from build123d import *

# Parameters (mm, degrees)
SKETCH1_W               = 49.5
SKETCH1_H               = 61.5
BOSS_EXTRUDE1_DEPTH     = 23.75
SKETCH2_W               = 46
SKETCH2_H               = 58
CUT_EXTRUDE1_DEPTH      = 22
SKETCH3_W               = 3
SKETCH3_H               = 16
CUT_EXTRUDE2_DEPTH      = 1.75
SKETCH7_W               = 3
SKETCH7_H               = 5
BOSS_EXTRUDE2_DEPTH     = 6
SKETCH11_W              = 37.5
SKETCH11_H              = 61.5
BOSS_EXTRUDE3_DEPTH     = 15
SKETCH12_W              = 34.5
SKETCH12_H              = 57
CUT_EXTRUDE3_DEPTH      = 15
SKETCH14_W              = 7.75
SKETCH14_H              = 9
BOSS_EXTRUDE4_DEPTH     = 0.0001
SKETCH15_W              = 4.15
SKETCH15_H              = 5.2
CUT_EXTRUDE4_DEPTH      = 4.75
SKETCH16_W              = 8.5
SKETCH16_H              = 15.5
BOSS_EXTRUDE5_DEPTH     = 16.75
SKETCH17_W              = 5.125
SKETCH17_H              = 6.625
CUT_EXTRUDE5_DEPTH      = 8.5
CUT_EXTRUDE6_DEPTH      = 15
CUT_EXTRUDE6_DEPTH_BACK = 1.75
SKETCH18_W              = 5
SKETCH18_H              = 12
SKETCH20_W              = 16
SKETCH20_H              = 4.5
CUT_EXTRUDE7_DEPTH      = 1.75
SKETCH21_W              = 32.25
SKETCH21_H              = 81.5
BOSS_EXTRUDE7_DEPTH     = 10
SKETCH23_W              = 28.75
SKETCH23_H              = 78
CUT_EXTRUDE8_DEPTH      = 10
SKETCH25_W              = 3
SKETCH25_H              = 5.4
BOSS_EXTRUDE8_DEPTH     = 1.75
SKETCH28_W              = 3
SKETCH28_H              = 2
BOSS_EXTRUDE9_DEPTH     = 1.75
SKETCH30_W              = 5
SKETCH30_H              = 1.5
BOSS_EXTRUDE11_DEPTH    = 1
SKETCH32_W              = 10.5
SKETCH32_H              = 2.25
CUT_EXTRUDE9_DEPTH      = 1.75
SKETCH33_W              = 11
SKETCH33_H              = 11
CUT_EXTRUDE10_DEPTH     = 1
SKETCH34_W              = 11
SKETCH34_H              = 1
BOSS_EXTRUDE12_DEPTH    = 2
SKETCH35_W              = 19
SKETCH35_H              = 10
CUT_EXTRUDE11_DEPTH     = 1.75
SKETCH36_W              = 1.75
SKETCH36_H              = 21.5
CUT_EXTRUDE12_DEPTH     = 5.75
SKETCH37_W              = 7.5
SKETCH37_H              = 7.5
SKETCH37_W_2            = 28.75
BOSS_EXTRUDE13_DEPTH    = 1.75


with BuildPart() as part:
    # Sketch1 → Boss-Extrude1 (new body)
    with BuildSketch(Plane(origin=(0, 0, 0), x_dir=(1, 0, 0), z_dir=(0, 1, 0))):
        with Locations((-113.412024913, -45.391200727)):
            Rectangle(SKETCH1_W, SKETCH1_H)
    extrude(amount=BOSS_EXTRUDE1_DEPTH)

    # Sketch2 → Cut-Extrude1 (cut)
    with BuildSketch(Plane(origin=(0, 0, 0), x_dir=(-1, 0, 0), z_dir=(0, -1, 0))):
        with Locations((113.412024913, -45.391200727)):
            Rectangle(SKETCH2_W, SKETCH2_H)
    extrude(amount=-CUT_EXTRUDE1_DEPTH, mode=Mode.SUBTRACT)

    # Sketch3 → Cut-Extrude2 (cut)
    with BuildSketch(Plane(origin=(0, 22, 0), x_dir=(-1, 0, 0), z_dir=(0, -1, 0))):
        with Locations((91.912024913, -66.391200727)):
            Rectangle(SKETCH3_W, SKETCH3_H)
        with Locations((91.912024913, -24.391200727)):
            Rectangle(SKETCH3_W, SKETCH3_H)
        with Locations((91.912024913, -45.391200727)):
            Rectangle(SKETCH3_W, SKETCH3_H)
    extrude(amount=-CUT_EXTRUDE2_DEPTH, mode=Mode.SUBTRACT)

    # Sketch7 → Boss-Extrude2 (add)
    with BuildSketch(Plane(origin=(0, 22, 0), x_dir=(-1, 0, 0), z_dir=(0, -1, 0))):
        with Locations((91.912024913, -55.891200727)):
            Rectangle(SKETCH7_W, SKETCH7_H)
        with Locations((91.912024913, -34.891200727)):
            Rectangle(SKETCH7_W, SKETCH7_H)
    extrude(amount=BOSS_EXTRUDE2_DEPTH)

    # Sketch11 → Boss-Extrude3 (add)
    with BuildSketch(Plane(origin=(0, 23.75, 0), x_dir=(1, 0, 0), z_dir=(0, 1, 0))):
        with Locations((-119.412024913, -45.391200727)):
            Rectangle(SKETCH11_W, SKETCH11_H)
    extrude(amount=BOSS_EXTRUDE3_DEPTH)

    # Sketch12 → Cut-Extrude3 (cut)
    with BuildSketch(Plane(origin=(0, 38.75, 0), x_dir=(1, 0, 0), z_dir=(0, 1, 0))):
        with Locations((-119.412024913, -45.391200727)):
            Rectangle(SKETCH12_W, SKETCH12_H)
    extrude(amount=-CUT_EXTRUDE3_DEPTH, mode=Mode.SUBTRACT)

    # Sketch14 → Boss-Extrude4 (add)
    with BuildSketch(Plane(origin=(0, 23.75, 0), x_dir=(1, 0, 0), z_dir=(0, 1, 0))):
        with Locations((-92.542024913, -66.391200727)):
            Rectangle(SKETCH14_W, SKETCH14_H)
    extrude(amount=BOSS_EXTRUDE4_DEPTH)

    # Sketch15 → Cut-Extrude4 (cut)
    with BuildSketch(Plane(origin=(0, 23.7501, 0), x_dir=(1, 0, 0), z_dir=(0, 1, 0))):
        with Locations((-92.542024913, -66.391200727)):
            Rectangle(SKETCH15_W, SKETCH15_H)
    extrude(amount=-CUT_EXTRUDE4_DEPTH, mode=Mode.SUBTRACT)

    # Sketch16 → Boss-Extrude5 (add)
    with BuildSketch(Plane(origin=(0, 23.75, 0), x_dir=(1, 0, 0), z_dir=(0, 1, 0))):
        with Locations((-92.912024913, -24.391200727)):
            Rectangle(SKETCH16_W, SKETCH16_H)
    extrude(amount=BOSS_EXTRUDE5_DEPTH)

    # Sketch17 → Cut-Extrude5 (cut)
    with BuildSketch(Plane(origin=(-88.662024913, 0, 0), x_dir=(0, 0, -1), z_dir=(1, 0, 0))):
        with Locations((-27.828700727, 35.4375)):
            Rectangle(SKETCH17_W, SKETCH17_H)
        with Locations((-27.828700727, 27.0625)):
            Rectangle(SKETCH17_W, SKETCH17_H)
        with Locations((-20.953700727, 35.4375)):
            Rectangle(SKETCH17_W, SKETCH17_H)
        with Locations((-20.953700727, 27.0625)):
            Rectangle(SKETCH17_W, SKETCH17_H)
    extrude(amount=-CUT_EXTRUDE5_DEPTH, mode=Mode.SUBTRACT)

    # Sketch18 → Cut-Extrude6 (cut, two sides: drawn at the far end of the back side and taken through both)
    with BuildSketch(Plane(origin=(0, 23.75, 0), x_dir=(1, 0, 0), z_dir=(0, 1, 0)).offset(-CUT_EXTRUDE6_DEPTH_BACK)):
        with Locations((-92.912024913, -24.391200727)):
            Rectangle(SKETCH18_W, SKETCH18_H)
    extrude(amount=CUT_EXTRUDE6_DEPTH + CUT_EXTRUDE6_DEPTH_BACK, mode=Mode.SUBTRACT)

    # Sketch20 → Cut-Extrude7 (cut)
    with BuildSketch(Plane(origin=(-100.662024913, 0, 0), x_dir=(0, 0, -1), z_dir=(1, 0, 0))):
        with Locations((-45.391200727, 26)):
            Rectangle(SKETCH20_W, SKETCH20_H)
    extrude(amount=-CUT_EXTRUDE7_DEPTH, mode=Mode.SUBTRACT)

    # Sketch21 → Boss-Extrude7 (add)
    with BuildSketch(Plane(origin=(0, 0, 0), x_dir=(-1, 0, 0), z_dir=(0, -1, 0))):
        with Locations((152.537024913, -45.391200727)):
            Rectangle(SKETCH21_W, SKETCH21_H)
    extrude(amount=-BOSS_EXTRUDE7_DEPTH)

    # Sketch23 → Cut-Extrude8 (cut)
    with BuildSketch(Plane(origin=(0, 10, 0), x_dir=(1, 0, 0), z_dir=(0, 1, 0))):
        with Locations((-152.537024913, -45.391200727)):
            Rectangle(SKETCH23_W, SKETCH23_H)
    extrude(amount=-CUT_EXTRUDE8_DEPTH, mode=Mode.SUBTRACT)

    # Sketch25 → Boss-Extrude8 (add)
    with BuildSketch(Plane(origin=(0, 22, 0), x_dir=(-1, 0, 0), z_dir=(0, -1, 0))):
        with Locations((91.912024913, -61.091200727)):
            Rectangle(SKETCH25_W, SKETCH25_H)
        with Locations((91.912024913, -71.691200727)):
            Rectangle(SKETCH25_W, SKETCH25_H)
    extrude(amount=-BOSS_EXTRUDE8_DEPTH)

    # Sketch28 → Boss-Extrude9 (add)
    with BuildSketch(Plane(origin=(0, 23.75, 0), x_dir=(1, 0, 0), z_dir=(0, 1, 0))):
        with Locations((-91.912024913, -17.391200727)):
            Rectangle(SKETCH28_W, SKETCH28_H)
        with Locations((-91.912024913, -31.391200727)):
            Rectangle(SKETCH28_W, SKETCH28_H)
    extrude(amount=-BOSS_EXTRUDE9_DEPTH)

    # Sketch30 → Boss-Extrude11 (add)
    with BuildSketch(Plane.ZY.offset(93.412024913)):
        with Locations((55.891200727, 16.75)):
            Rectangle(SKETCH30_W, SKETCH30_H)
        with Locations((34.891200727, 16.75)):
            Rectangle(SKETCH30_W, SKETCH30_H)
    extrude(amount=BOSS_EXTRUDE11_DEPTH)

    # Sketch32 → Cut-Extrude9 (cut)
    with BuildSketch(Plane(origin=(0, 38.75, 0), x_dir=(1, 0, 0), z_dir=(0, 1, 0))):
        with Locations((-119.412024913, -75.016200727)):
            Rectangle(SKETCH32_W, SKETCH32_H)
        with Locations((-119.412024913, -15.766200727)):
            Rectangle(SKETCH32_W, SKETCH32_H)
    extrude(amount=-CUT_EXTRUDE9_DEPTH, mode=Mode.SUBTRACT)

    # Sketch33 → Cut-Extrude10 (cut)
    with BuildSketch(Plane.ZY.offset(90.412024913)):
        with Locations((32.891200727, 5.5)):
            Rectangle(SKETCH33_W, SKETCH33_H)
    extrude(amount=-CUT_EXTRUDE10_DEPTH, mode=Mode.SUBTRACT)

    # Sketch34 → Boss-Extrude12 (add)
    with BuildSketch(Plane.ZY.offset(90.412024913)):
        with Locations((32.891200727, 11.5)):
            Rectangle(SKETCH34_W, SKETCH34_H)
        Polygon((38.391200727, 12), (38.391200727, 11), (38.391200727, 0), (39.391200727, 0), (39.391200727, 12), align=None)
        Polygon((26.391200727, 0), (27.391200727, 0), (27.391200727, 11), (27.391200727, 12), (26.391200727, 12), align=None)
    extrude(amount=BOSS_EXTRUDE12_DEPTH)

    # Sketch35 → Cut-Extrude11 (cut)
    with BuildSketch(Plane(origin=(0, 0, 14.641200727), x_dir=(-1, 0, 0), z_dir=(0, 0, -1))):
        with Locations((123.412024913, 5)):
            Rectangle(SKETCH35_W, SKETCH35_H)
    extrude(amount=-CUT_EXTRUDE11_DEPTH, mode=Mode.SUBTRACT)

    # Sketch36 → Cut-Extrude12 (cut)
    with BuildSketch(Plane(origin=(0, 0, 0), x_dir=(-1, 0, 0), z_dir=(0, -1, 0))):
        with Locations((137.287024913, -45.391200727)):
            Rectangle(SKETCH36_W, SKETCH36_H)
    extrude(amount=-CUT_EXTRUDE12_DEPTH, mode=Mode.SUBTRACT)

    # Sketch37 → Boss-Extrude13 (add)
    with BuildSketch(Plane(origin=(0, 0, 0), x_dir=(-1, 0, 0), z_dir=(0, -1, 0))):
        with Locations((94.162024913, -70.641200727)):
            Rectangle(SKETCH37_W, SKETCH37_H)
        with Locations((94.162024913, -20.141200727)):
            Rectangle(SKETCH37_W, SKETCH37_H)
        with Locations((152.537024913, -70.641200727)):
            Rectangle(SKETCH37_W_2, SKETCH37_H)
        with Locations((152.537024913, -20.141200727)):
            Rectangle(SKETCH37_W_2, SKETCH37_H)
    extrude(amount=-BOSS_EXTRUDE13_DEPTH)


solid = part.part
For this review, take the finished solid that the model builds, in its own axes (mm). A direction names the side the tool comes from. Give positions to 0.01 mm unless a question says otherwise; leave off trailing zeros. Order: outer loops, then holes, each group sorted by start corner. A loop starts at its lowest first (then second) coordinate and runs counter-clockwise, first axis right, second up. Notation, with made-up numbers: (12, -29.75) - (49, -29.75) arc R11 cw to (49, -24.75) - close; hole circle Ø7 at (-37, 64). An arc over 180 degrees is marked (long way). Answer as a JSON object with one key per item and string values. Group by question number.
Item 1: Clearance check with flat-ended pins moving along their axes: pin 1 Ø4.5 at (y, z) = (30.5, 26.5) entering from -X; pin 2 Ø3 at (x, z) = (-126, 22.5) entering from +Y; pin 3 Ø12 at (x, z) = (-137, 67.5) entering from +Y. State where each tip first meets the part, or that it passes through.
Item 2: Take a section at C-C on z = 45. Give the boundary of the cut face in (x, y).
Item 3: Wall thickness on line 1 along X through (y, z) = (8, 36); line 2 along X through (y, z) = (2, 60.5); line 3 along Y through (x, z) = (-97, 21.5) (3 decimals): over which ranges is each line inside the solid? List them lowest first.
Item 4: Take a section at B-B on y = 26. Give the boundary of the cut face in (x, z).
Item 5: Machinability: for faces 4 (the flat face through (-89.412, 6, 33)), 5 (the flat face through (-95, 23.75, 66)), 6 (the flat face through (-102, 38.75, 45)), which of the approach directions +Z, -Z, +X, -X, +Y, -Y give a long, thin tool a straight path to every point of the face, cutting with its end or side? Answer none if there is none.
Item 6: Take a section at A-A on y = 35. Give the boundary of the cut face in (x, z), and give its area (3 significant figures).
Item 7: Draft analysis for pull direction Y (two halves, no side actions). For faces 1 (the flat face through (-92, 19, 32.391)), 2 (the flat face through (-136.412, 11, 46)), 3 (the flat face through (-137, 0, 60)), state which applies: pulls with the +Y half, pulls with the -Y half, needs draft (parallel to the pull), parting line crosses it, or undercut.
Item 8: Take a section at D-D on x = -156. Give the boundary of the cut face in (y, z).
Reported:
{
 "1": {"pin 1": "x = -138.16", "pin 2": "y = 23.75", "pin 3": "y = 38.75"},
 "2": {"outline": "(-168.66, 0) - (-166.91, 0) - (-166.91, 10) - (-168.66, 10) - close; (-138.16, 5.75) - (-136.41, 5.75) - (-136.41, 22) - (-93.41, 22) - (-93.41, 23.75) - (-136.66, 23.75) - (-136.66, 38.75) - (-138.16, 38.75) - close; (-102.16, 28.25) - (-100.66, 28.25) - (-100.66, 38.75) - (-102.16, 38.75) - close; (-90.41, 0) - (-88.66, 0) - (-88.66, 23.75) - (-90.41, 23.75) - close"},
 "3": {"line 1": "-168.66 to -166.91, -138.16 to -136.41, -89.41 to -88.66", "line 2": "-168.66 to -166.91, -138.16 to -136.41, -90.41 to -88.66", "line 3": "0 to 1.75, 22 to 23.75, 30.375 to 32.125, 38.75 to 40.5"},
 "4": {"outline": "(-138.16, 14.64) - (-100.66, 14.64) - (-100.66, 37.39) - (-102.16, 37.39) - (-102.16, 16.89) - (-136.66, 16.89) - (-136.66, 73.89) - (-102.16, 73.89) - (-102.16, 53.39) - (-100.66, 53.39) - (-100.66, 76.14) - (-138.16, 76.14) - close; (-97.16, 16.64) - (-88.66, 16.64) - (-88.66, 18.39) - (-97.16, 18.39) - close; (-97.16, 23.52) - (-95.41, 23.52) - (-95.41, 25.27) - (-97.16, 25.27) - close; (-97.16, 30.39) - (-88.66, 30.39) - (-88.66, 32.14) - (-97.16, 32.14) - close; (-90.41, 23.52) - (-88.66, 23.52) - (-88.66, 25.27) - (-90.41, 25.27) - close"},
 "5": {"face 4": "-Y", "face 5": "+Z, +X, +Y", "face 6": "+Z, -Z, -X, +Y"},
 "6": {"outline": "(-138.16, 14.64) - (-100.66, 14.64) - (-100.66, 76.14) - (-138.16, 76.14) - close; (-97.16, 16.64) - (-88.66, 16.64) - (-88.66, 18.39) - (-97.16, 18.39) - close; (-97.16, 23.52) - (-95.41, 23.52) - (-95.41, 25.27) - (-97.16, 25.27) - close; (-97.16, 30.39) - (-88.66, 30.39) - (-88.66, 32.14) - (-97.16, 32.14) - close; (-90.41, 23.52) - (-88.66, 23.52) - (-88.66, 25.27) - (-90.41, 25.27) - close; hole (-136.66, 16.89) - (-102.16, 16.89) - (-102.16, 73.89) - (-136.66, 73.89) - close", "area": "376 mm^2"},
 "7": {"face 1": "undercut", "face 2": "needs draft", "face 3": "pulls with the -Y half"},
 "8": {"outline": "(0, 4.64) - (10, 4.64) - (10, 6.39) - (0, 6.39) - close; (0, 16.39) - (1.75, 16.39) - (1.75, 23.89) - (0, 23.89) - close; (0, 66.89) - (1.75, 66.89) - (1.75, 74.39) - (0, 74.39) - close; (0, 84.39) - (10, 84.39) - (10, 86.14) - (0, 86.14) - close"}
}
